from build123d import *

# Parameters (mm, degrees)
F0_W     = 506
F0_H     = 241
F0_R     = 111
F0_R_2   = 94.5
F1_DEPTH = 12


with BuildPart() as f1:
    # F0 (on Front) → F1 (new body)
    with BuildSketch(Plane.XZ):
        Rectangle(F0_W, F0_H)
        with Locations((-121, 0)):
            Circle(F0_R, mode=Mode.SUBTRACT)
        with Locations((121, 0)):
            Circle(F0_R, mode=Mode.SUBTRACT)
        with Locations((-121, 0)):
            Circle(F0_R)
        with Locations((-121, 0)):
            Circle(F0_R_2, mode=Mode.SUBTRACT)
        with Locations((121, 0)):
            Circle(F0_R)
        with Locations((121, 0)):
            Circle(F0_R_2, mode=Mode.SUBTRACT)
    extrude(amount=F1_DEPTH)


solid = f1.part
Read the model definition and answer for the solid it produces. Units are mm, in the model's axes. Give positions to 0.01 mm unless a question says otherwise; leave off trailing zeros. Write each loop counter-clockwise with the first axis right and the second up, starting at its lowest first coordinate (ties: lowest second). Pieces come first, ordered by that corner, then holes. Notation, with made-up numbers: M -35,84.25 L -18,84.25 A17 ccw -18,96.25 Z; hole C 30.5,57.25 d4. An arc over 180 degrees is marked long. One line per item, written item: value. Start each with the question number.
(1) Determine the mould class of faces 1 (the cylindrical face through (208.294, -5.916, -36.194)), 2 (the flat face through (-4, 0, 2)), 3 (the flat face through (-4, -6, -120.5)) for opening direction Z: pulls with the +Z half, pulls with the -Z half, needs draft (parallel to the pull), parting line crosses it, or undercut.
(2) Find section B-B (z = 0). Determine the outline of the cut face in (x, y).
(3) Find section A-A (x = -121). Determine the outline of the cut face in (y, z), plus the area to 3 significant figures.
(4) Find the intervals of material crossed by line 1 (Z direction, x = 121.5, y = -0.75); line 2 (X direction, y = -6.5, z = -21); line 3 (X direction, y = -6.5, z = 57.5), in increasing order.
(5) Find section C-C (y = -6.25). Determine the outline of the cut face in (x, z).
(6) Find section D-D (x = 161). Determine the outline of the cut face in (y, z).
Results below:
1. face 1: undercut
1. face 2: needs draft
1. face 3: pulls with the -Z half
2. outline: M -253,-12 L -215.5,-12 L -215.5,0 L -253,0 Z; M -26.5,-12 L 26.5,-12 L 26.5,0 L -26.5,0 Z; M 215.5,-12 L 253,-12 L 253,0 L 215.5,0 Z
3. outline: M -12,-120.5 L 0,-120.5 L 0,-94.5 L -12,-94.5 Z; M -12,94.5 L 0,94.5 L 0,120.5 L -12,120.5 Z
3. area: 624 mm^2
4. line 1: z = -120.5 to -94.5, 94.5 to 120.5
4. line 2: x = -253 to -213.14, -28.86 to 28.86, 213.14 to 253
4. line 3: x = -253 to -195.99, -46.01 to 46.01, 195.99 to 253
5. outline: M -253,-120.5 L 253,-120.5 L 253,120.5 L -253,120.5 Z; hole C -121,0 d189; hole C 121,0 d189
6. outline: M -12,-120.5 L 0,-120.5 L 0,-85.62 L -12,-85.62 Z; M -12,85.62 L 0,85.62 L 0,120.5 L -12,120.5 Z
